Answer from the drawing. Dimensions are ordinates in mm from the lowest x, y and z of the part. A direction names the side the tool comes from. Coordinates: 2 decimals unless noted, no trailing zeros. Order: outer loops, then holes, each group sorted by start corner. A loop starts at its lowest first (then second) coordinate and runs counter-clockwise, first axis right, second up. Notation, with made-up numbers: (49.5, 38) -> (95.5, 38) arc R34 cw to (95.5, 71) -> close; hole circle Ø2 at (-24, 86.5). An arc over 180 degrees is marked (long way). Use CSV: the item, a comma, the result in double quotes.
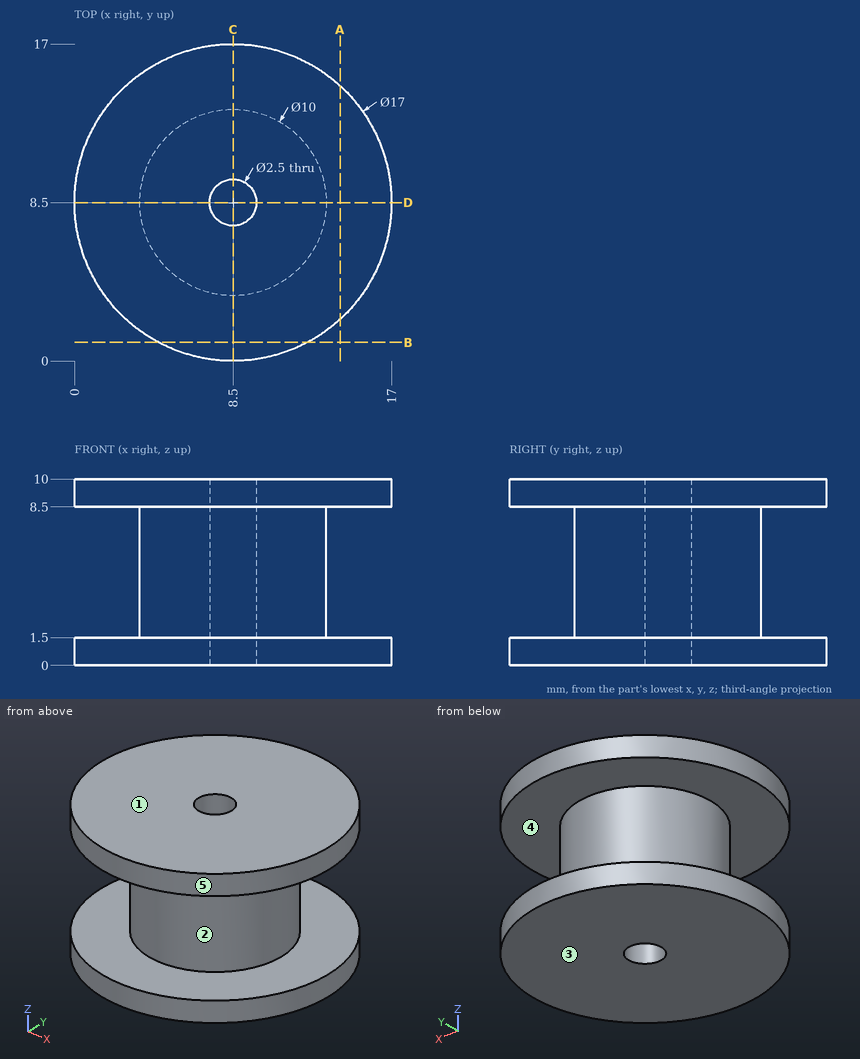
Item 1: The mould has two halves that part along Z. Classify the marked faces 3, 4 and 5: +Z half, -Z half, draft (parallel to the pull), parting line (faces both ways), or undercut.
Return value:
face 3,"-Z half"
face 4,"undercut"
face 5,"draft"
Item 2: Straight lines are drawn through the part: line 1 along Z through (x, y) = (9.5, 13.5); line 2 along Y through (x, z) = (8.5, 3); line 3 along X through (y, z) = (7.5, 6). For each, find the intervals that lie inside material, in ascending order.
Return value:
line 1,"z = 0 to 1.5, 8.5 to 10"
line 2,"y = 3.5 to 7.25, 9.75 to 13.5"
line 3,"x = 3.6 to 7.75, 9.25 to 13.4"
Item 3: Find section B-B, the plane y = 1. Give the vertices of the cut face in (x, z).
Return value:
outline,"(4.5, 0) -> (12.5, 0) -> (12.5, 1.5) -> (4.5, 1.5) -> close; (4.5, 8.5) -> (12.5, 8.5) -> (12.5, 10) -> (4.5, 10) -> close"
Item 4: Find section C-C, the plane x = 8.5. Give the vertices of the cut face in (y, z).
Return value:
outline,"(0, 0) -> (7.25, 0) -> (7.25, 10) -> (0, 10) -> (0, 8.5) -> (3.5, 8.5) -> (3.5, 1.5) -> (0, 1.5) -> close; (9.75, 0) -> (17, 0) -> (17, 1.5) -> (13.5, 1.5) -> (13.5, 8.5) -> (17, 8.5) -> (17, 10) -> (9.75, 10) -> close"
Item 5: Each of these flat-tipped pins is pushed along its axis until it touches: P1, Ø1.5, axis at y = 8.5, z = 4, coming from the +X side; P2, Ø2, axis at x = 5, z = 7, coming from the +Y side; P3, Ø2, axis at x = 12.5, z = 4.5, coming from the -Y side. Where does it stop, or does it pass through?
Return value:
P1,"stops at x = 13.5"
P2,"stops at y = 12.83"
P3,"stops at y = 4.5"
Item 6: A tool of negligible diameter and unlimited length cuts with its end or side. For the marked faces 1 and 2, from which of +Z, -Z, +X, -X, +Y, -Y can it reach the whole face along a straight path? Write none if from no direction.
Return value:
face 1,"+Z, +X, -X, +Y, -Y"
face 2,"none"
Item 7: Find section A-A, the plane x = 14.25. Give the vertices of the cut face in (y, z).
Return value:
outline,"(2.24, 0) -> (14.76, 0) -> (14.76, 1.5) -> (2.24, 1.5) -> close; (2.24, 8.5) -> (14.76, 8.5) -> (14.76, 10) -> (2.24, 10) -> close"
